```python
from build123d import *

# Parameters (mm, degrees)
F3_W     = 140
F3_H     = 140
F4_DEPTH = 20
F0_W     = 15.1
F0_H     = 14
F6_START = 14
F6_DEPTH = 136
F7_START = 19
F7_DEPTH = 6


with BuildPart() as f4:
    # F3 (on Top) → F4 (new body)
    with BuildSketch(Plane.XY):
        Rectangle(F3_W, F3_H)
    extrude(amount=F4_DEPTH)

    # F0 (on Front) → F5 (revolve, cut)
    with BuildSketch(Plane.XZ):
        with Locations((7.55, 13)):
            Rectangle(F0_W, F0_H)
    revolve(axis=Axis((0, 0, 13), (0, 0, -1)), mode=Mode.SUBTRACT)

    # F1 (on Right) → F6 (cut)
    with BuildSketch(Plane.YZ.offset(F6_START)):
        with BuildLine():
            Line((4.5, 20.4638522118), (0, 20.4638522118))
            Line((0, 20.4638522118), (-4.5, 20.4638522118))
            Line((-4.5, 20.4638522118), (-4.5, 10.4638522118))
            ThreePointArc((-4.5, 10.4638522118), (0, 5.9638522118), (4.5, 10.4638522118))
            Line((4.5, 10.4638522118), (4.5, 20.4638522118))
        make_face()
    extrude(amount=F6_DEPTH, mode=Mode.SUBTRACT)

    # F2 (on Top) → F7 (cut)
    with BuildSketch(Plane.XY.offset(F7_START)):
        Polygon((14, 0.5), (14, 0), (14, -0.5), (74, -0.5), (74, 0.5), align=None)
        Polygon((0.5, -14), (0, -14), (-0.5, -14), (-0.5, -74), (0.5, -74), align=None)
        Polygon((-13.9910685796, -0.5), (-13.9910685796, 0), (-13.9910685796, 0.5), (-73.9910685796, 0.5), (-73.9910685796, -0.5), align=None)
        Polygon((-0.5, 73.9972595498), (-0.5, 13.9972595498), (0, 13.9972595498), (0.5, 13.9972595498), (0.5, 73.9972595498), align=None)
    extrude(amount=F7_DEPTH, mode=Mode.SUBTRACT)


solid = f4.part
```
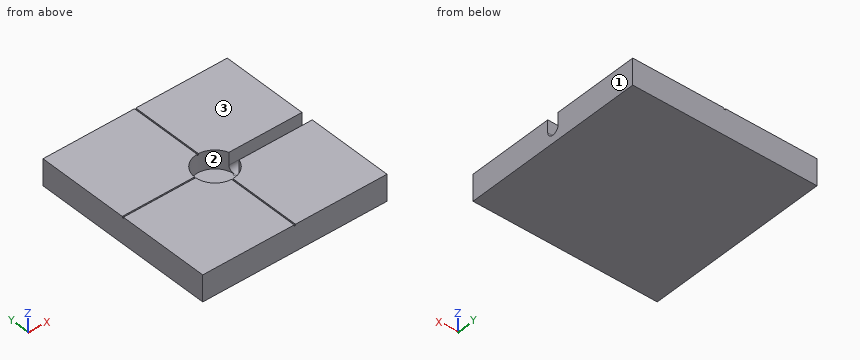
Design review of the part built by this model. Coordinates are the model's own, in mm. Face numbers are marked on the shaded views. Coordinates: 2 decimals unless noted, no trailing zeros. Order: outer loops, then holes, each group sorted by start corner. A loop starts at its lowest first (then second) coordinate and runs counter-clockwise, first axis right, second up. Notation, with made-up numbers: M -23,49.5 L 32,49.5 A20 ccw 32,62.5 Z; hole C -33,5 d9. An arc over 180 degrees is marked long. Answer as a JSON object with one key per item and string values. Group by question number.
1) Wall thickness on L1, parallel to Y at x = 0, z = 15.25; L2, parallel to Y at x = 17, z = 12.75; L3, parallel to X at y = 0, z = 12.5: over which ranges is each line inside the solid? List them lowest first.
2) Add section A-A, the plane z = 16. Write out the cut boundary in (x, y), then the cut area to 3 significant figures.
3) Mouldability with a two-part tool opening along X and no side actions: class the marked faces 1, 2 and 3 as pulls with the +X half, pulls with the -X half, needs draft (parallel to the pull), parting line crosses it, or undercut.
4) For pin 1 (0.8 mm diameter, centred on x = 0, y = -38, fed in from +Z), flat-tipped, find the tip position at first contact; note if it passes through.
5) Add section B-B, the plane x = -12.5. Write out the cut boundary in (y, z).
Computed values:
{
 "1": {"L1": "y = -70 to -15.1, 15.1 to 70", "L2": "y = -70 to -4.5, 4.5 to 70", "L3": "x = -70 to -15.1"},
 "2": {"outline": "M -70,-70 L 70,-70 L 70,-4.5 L 14.41,-4.5 A15.1 cw long 14.41,4.5 L 70,4.5 L 70,70 L -70,70 Z", "area": "18,400 mm^2"},
 "3": {"face 1": "pulls with the +X half", "face 2": "undercut", "face 3": "needs draft"},
 "4": {"pin 1": "stops at z = 19"},
 "5": {"outline": "M -70,0 L 70,0 L 70,20 L 8.47,20 L 8.47,6 L -8.47,6 L -8.47,20 L -70,20 Z"}
}
